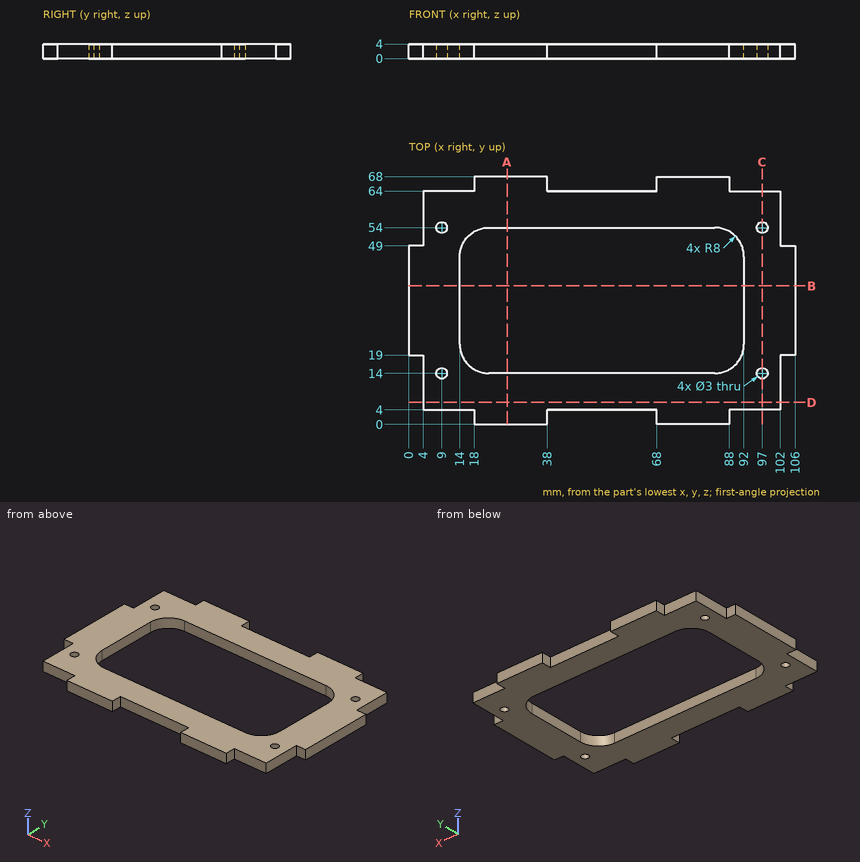
Drawing for the job (mm, zero at the part's lowest x, y, z). Round coordinates to 2 decimals unless told otherwise and drop trailing zeros. Order: outer loops, then holes, each group sorted by start corner. A loop starts at its lowest first (then second) coordinate and runs counter-clockwise, first axis right, second up.
Item 1: Saw through at C-C on x = 97. Write the cut outline in (y, z), then the cut area to 3 significant figures.
Item 2: Pin check, flat tips, straight feed: pin 1 (2 mm diameter, centred on y = 14.5, z = 1.5, fed in from -X); pin 2 (2 mm diameter, centred on x = 103.5, z = 2, fed in from -Y); pin 3 (1.2 mm diameter, centred on y = 1.5, z = 2.5, fed in from -X). Stop position of each tip, or through.
Item 3: Saw through at A-A on x = 27. Write the cut outline in (y, z), then the cut area to 3 significant figures.
Item 4: Saw through at B-B on y = 38. Write the cut outline in (x, z), then the cut area to 3 significant figures.
Item 5: Saw through at D-D on y = 6. Write the cut outline in (x, z), then the cut area to 3 significant figures.
Item 6: Probe line 1 along Y through (x, z) = (9, 1.6); line 2 along Y through (x, z) = (31.5, 2.9); line 3 along Y through (x, z) = (66, 2.6). List the from-to ranges inside material, lowest first.
Reported:
1. outline: (4, 0) - (12.5, 0) - (12.5, 4) - (4, 4) - close; (15.5, 0) - (52.5, 0) - (52.5, 4) - (15.5, 4) - close; (55.5, 0) - (64, 0) - (64, 4) - (55.5, 4) - close
1. area: 216 mm2
2. pin 1: stops at x = 4
2. pin 2: stops at y = 19
2. pin 3: stops at x = 18
3. outline: (0, 0) - (14, 0) - (14, 4) - (0, 4) - close; (54, 0) - (68, 0) - (68, 4) - (54, 4) - close
3. area: 112 mm2
4. outline: (0, 0) - (14, 0) - (14, 4) - (0, 4) - close; (92, 0) - (106, 0) - (106, 4) - (92, 4) - close
4. area: 112 mm2
5. outline: (4, 0) - (102, 0) - (102, 4) - (4, 4) - close
5. area: 392 mm2
6. line 1: y = 4 to 12.5, 15.5 to 52.5, 55.5 to 64
6. line 2: y = 0 to 14, 54 to 68
6. line 3: y = 4 to 14, 54 to 64
